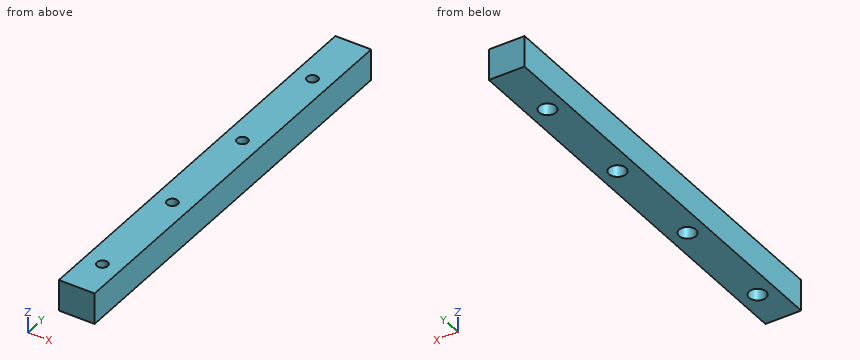
```python
from build123d import *

# Parameters (mm, degrees)
SKETCH_1_W          = 20
SKETCH_1_H          = 17.5
EXTRUDE_1_DEPTH     = 237
SKETCH_2_R          = 3
CUT_EXTRUDE_1_DEPTH = 238.855523375
CUT_EXTRUDE_START   = -17.5
SKETCH_3_R          = 4.75
CUT_EXTRUDE_2_DEPTH = 8.5


with BuildPart() as part:
    # 草图1 → 凸台-拉伸1 (new body)
    with BuildSketch(Plane(origin=(0, 0, 0), x_dir=(1, 0, 0), z_dir=(0, 1, 0))):
        with Locations((0, 8.75)):
            Rectangle(SKETCH_1_W, SKETCH_1_H)
    extrude(amount=EXTRUDE_1_DEPTH)

    # 草图2 → 切除-拉伸1 (cut, through all)
    with BuildSketch(Plane.XY):
        with Locations((0, 22)):
            Circle(SKETCH_2_R)
        with Locations((0, 82)):
            Circle(SKETCH_2_R)
        with Locations((0, 142)):
            Circle(SKETCH_2_R)
        with Locations((0, 202)):
            Circle(SKETCH_2_R)
        with Locations((0, 262)):
            Circle(SKETCH_2_R)
    extrude(amount=-CUT_EXTRUDE_1_DEPTH, mode=Mode.SUBTRACT)

    # 草图3 → 切除-拉伸2 (cut)
    with BuildSketch(Plane.XY.offset(CUT_EXTRUDE_START)):
        with Locations((0, 22)):
            Circle(SKETCH_3_R)
        with Locations((0, 82)):
            Circle(SKETCH_3_R)
        with Locations((0, 142)):
            Circle(SKETCH_3_R)
        with Locations((0, 202)):
            Circle(SKETCH_3_R)
        with Locations((0, 262)):
            Circle(SKETCH_3_R)
    extrude(amount=CUT_EXTRUDE_2_DEPTH, mode=Mode.SUBTRACT)


solid = part.part
```
Model file for the job. Use its own axes, mm. Coordinates: 2 decimals unless noted, no trailing zeros. Loops run counter-clockwise (first coordinate to the right, second up) from the corner with the lowest first, then second, coordinate; pieces in that order, holes last. Notation, with made-up numbers: (-22.75, 21.5) -> (2.25, 21.5) arc R21 ccw to (2.25, 60.5) -> close; hole circle Ø5 at (83, -30.75). An arc over 180 degrees is marked (long way). Answer as a JSON object with one key per item and string values.
Q1. Probe probe 1 along Y at (x, z) = (0, -2.5); probe 2 along Y at (x, z) = (0, -13.25); probe 3 along X at (y, z) = (142, -5.25). List the from-to ranges inside material, lowest first.
Report:
{"probe 1": "y = 0 to 19, 25 to 79, 85 to 139, 145 to 199, 205 to 237", "probe 2": "y = 0 to 17.25, 26.75 to 77.25, 86.75 to 137.25, 146.75 to 197.25, 206.75 to 237", "probe 3": "x = -10 to -3, 3 to 10"}
Q2. Flat gauge pin, fed straight in: P1, Ø7.5, axis at x = 0, y = 142, coming from the -Z side. Where does the tip first touch, or does it go through?
Report:
{"P1": "stops at z = -9"}
Q3. Cut at A-A (z = -2). List the corners of the cut face in (x, y).
Report:
{"outline": "(-10, 0) -> (10, 0) -> (10, 237) -> (-10, 237) -> close; hole circle Ø6 at (0, 22); hole circle Ø6 at (0, 82); hole circle Ø6 at (0, 142); hole circle Ø6 at (0, 202)"}
Q4. Cut at C-C (z = -14.25). List the corners of the cut face in (x, y).
Report:
{"outline": "(-10, 0) -> (10, 0) -> (10, 237) -> (-10, 237) -> close; hole circle Ø9.5 at (0, 22); hole circle Ø9.5 at (0, 82); hole circle Ø9.5 at (0, 142); hole circle Ø9.5 at (0, 202)"}
Q5. Cut at B-B (y = 22). List the corners of the cut face in (x, z), and give its area (3 significant figures).
Report:
{"outline": "(-10, -17.5) -> (-4.75, -17.5) -> (-4.75, -9) -> (-3, -9) -> (-3, 0) -> (-10, 0) -> close; (3, -9) -> (4.75, -9) -> (4.75, -17.5) -> (10, -17.5) -> (10, 0) -> (3, 0) -> close", "area": "215 mm2"}
